from build123d import *

# Parameters (mm, degrees)
SKETCH1_W           = 76.2
SKETCH1_H           = 203.2
BOSS_EXTRUDE1_DEPTH = 6.35
SKETCH6_R           = 1.778
CUT_EXTRUDE4_DEPTH  = 6.35
SKETCH7_W           = 21.336
SKETCH7_H           = 38.1
BOSS_EXTRUDE2_DEPTH = 8.754615714
SKETCH8_R           = 1.778
CUT_EXTRUDE5_DEPTH  = 218.542707108
SKETCH9_W           = 44.45
SKETCH9_H           = 139.7
CUT_EXTRUDE6_DEPTH  = 3.175
CHAMFER1_SIZE       = 10


with BuildPart() as part:
    # Sketch1 → Boss-Extrude1 (new body)
    with BuildSketch(Plane.XY):
        with Locations((38.1, 101.6)):
            Rectangle(SKETCH1_W, SKETCH1_H)
    extrude(amount=BOSS_EXTRUDE1_DEPTH)

    # Sketch6 → Cut-Extrude4 (cut)
    with BuildSketch(Plane(origin=(0, 0, 0), x_dir=(-1, 0, 0), z_dir=(0, 0, -1))):
        with Locations((-63.5, 6.35)):
            Circle(SKETCH6_R)
        with Locations((-12.7, 6.35)):
            Circle(SKETCH6_R)
        with Locations((-6.35, 177.8)):
            Circle(SKETCH6_R)
        with Locations((-6.35, 25.4)):
            Circle(SKETCH6_R)
        with Locations((-69.85, 25.4)):
            Circle(SKETCH6_R)
        with Locations((-69.85, 177.8)):
            Circle(SKETCH6_R)
        with Locations((-63.5, 196.85)):
            Circle(SKETCH6_R)
        with Locations((-12.7, 196.85)):
            Circle(SKETCH6_R)
        with Locations((-6.35, 101.6)):
            Circle(SKETCH6_R)
        with Locations((-69.85, 101.6)):
            Circle(SKETCH6_R)
    extrude(amount=-CUT_EXTRUDE4_DEPTH, mode=Mode.SUBTRACT)

    # Sketch7 → Boss-Extrude2 (add)
    with BuildSketch(Plane.XY.offset(6.35)):
        with Locations((38.1, 19.05)):
            Rectangle(SKETCH7_W, SKETCH7_H)
    extrude(amount=BOSS_EXTRUDE2_DEPTH)

    # Sketch8 → Cut-Extrude5 (cut, through all)
    with BuildSketch(Plane.XY.offset(15.104615714)):
        with Locations((34.1503, 5.5753)):
            Circle(SKETCH8_R)
        with Locations((42.0497, 5.5753)):
            Circle(SKETCH8_R)
        with Locations((42.0497, 32.5247)):
            Circle(SKETCH8_R)
        with Locations((34.1503, 32.5247)):
            Circle(SKETCH8_R)
        with Locations((38.1, 19.05)):
            Circle(SKETCH8_R)
    extrude(amount=-CUT_EXTRUDE5_DEPTH, mode=Mode.SUBTRACT)

    # Sketch9 → Cut-Extrude6 (cut)
    with BuildSketch(Plane.XY.offset(6.35)):
        with Locations((38.1, 120.65)):
            Rectangle(SKETCH9_W, SKETCH9_H)
    extrude(amount=-CUT_EXTRUDE6_DEPTH, mode=Mode.SUBTRACT)

    # Chamfer1
    # the kernel refuses this chamfer: 10 mm, written as the material it adds along each edge
    with BuildSketch(Plane(origin=(27.432, 38.1, 6.35), x_dir=(-0.9996219169112968, 0, -0.027495876610586403), z_dir=(0, -1, 0))) as chamfer1_piece_1_section:
        Polygon((CHAMFER1_SIZE * 0.999621916911, -CHAMFER1_SIZE * 0.0274958766106), (-CHAMFER1_SIZE * 0.0274958766106, -CHAMFER1_SIZE * 0.999621916911), (0, 0), align=None)
    chamfer1_piece_1 = extrude(amount=38.1, mode=Mode.PRIVATE)
    chamfer1_piece_1 = split(chamfer1_piece_1, bisect_by=Plane(origin=(24.052510744, 19.05, 15.104615714), z_dir=(0, 0, -1)), keep=Keep.TOP, mode=Mode.PRIVATE)
    add(chamfer1_piece_1)
    with BuildSketch(Plane(origin=(48.768, 38.1, 6.35), x_dir=(0, 0.9996219169112968, -0.027495876610586403), z_dir=(-1, 0, 0))) as chamfer1_piece_2_section:
        Polygon((CHAMFER1_SIZE * 0.999621916911, -CHAMFER1_SIZE * 0.0274958766106), (-CHAMFER1_SIZE * 0.0274958766106, -CHAMFER1_SIZE * 0.999621916911), (0, 0), align=None)
    chamfer1_piece_2 = extrude(amount=21.336, mode=Mode.PRIVATE)
    chamfer1_piece_2 = split(chamfer1_piece_2, bisect_by=Plane(origin=(38.1, 41.479489256, 15.104615714), z_dir=(0, 0, -1)), keep=Keep.TOP, mode=Mode.PRIVATE)
    add(chamfer1_piece_2)
    with BuildSketch(Plane(origin=(48.768, 0, 6.35), x_dir=(0.9996219169112968, 0, -0.027495876610586403), z_dir=(0, 1, 0))) as chamfer1_piece_3_section:
        Polygon((CHAMFER1_SIZE * 0.999621916911, -CHAMFER1_SIZE * 0.0274958766106), (-CHAMFER1_SIZE * 0.0274958766106, -CHAMFER1_SIZE * 0.999621916911), (0, 0), align=None)
    chamfer1_piece_3 = extrude(amount=38.1, mode=Mode.PRIVATE)
    chamfer1_piece_3 = split(chamfer1_piece_3, bisect_by=Plane(origin=(52.147489256, 19.05, 15.104615714), z_dir=(0, 0, -1)), keep=Keep.TOP, mode=Mode.PRIVATE)
    add(chamfer1_piece_3)
    with BuildSketch(Plane(origin=(27.432, 63.81682988, 6.35), x_dir=(-0.9996219169112968, 0, -0.027495876610586403), z_dir=(0, -1, 0))) as chamfer1_piece_4a_section:
        Polygon((CHAMFER1_SIZE * 0.999621916911, -CHAMFER1_SIZE * 0.0274958766106), (-CHAMFER1_SIZE * 0.0274958766106, -CHAMFER1_SIZE * 0.999621916911), (0, 0), align=None)
    chamfer1_piece_4a = extrude(amount=63.81682988, mode=Mode.PRIVATE)
    chamfer1_piece_4a = split(chamfer1_piece_4a, bisect_by=Plane(origin=(24.052510744, 50.8, 9.492641484), z_dir=(0, -1, 0)), keep=Keep.TOP, mode=Mode.PRIVATE)
    chamfer1_piece_4a = split(chamfer1_piece_4a, bisect_by=Plane(origin=(24.052510744, 38.1, 9.492641484), z_dir=(0, 1, 0)), keep=Keep.TOP, mode=Mode.PRIVATE)
    chamfer1_piece_4a = split(chamfer1_piece_4a, bisect_by=Plane(origin=(24.052510744, 44.45, 15.104615714), z_dir=(0, 0, -1)), keep=Keep.TOP, mode=Mode.PRIVATE)
    with BuildSketch(Plane(origin=(48.768, 38.1, 6.35), x_dir=(0, 0.9996219169112968, -0.027495876610586403), z_dir=(-1, 0, 0))) as chamfer1_piece_4b_section:
        Polygon((CHAMFER1_SIZE * 0.999621916911, -CHAMFER1_SIZE * 0.0274958766106), (-CHAMFER1_SIZE * 0.0274958766106, -CHAMFER1_SIZE * 0.999621916911), (0, 0), align=None)
    chamfer1_piece_4b = extrude(amount=47.05282988, mode=Mode.PRIVATE)
    chamfer1_piece_4b = split(chamfer1_piece_4b, bisect_by=Plane(origin=(27.432, 41.479489256, 9.492641484), z_dir=(-1, 0, 0)), keep=Keep.TOP, mode=Mode.PRIVATE)
    chamfer1_piece_4b = split(chamfer1_piece_4b, bisect_by=Plane(origin=(14.57358506, 41.479489256, 15.104615714), z_dir=(0, 0, -1)), keep=Keep.TOP, mode=Mode.PRIVATE)
    chamfer1_piece_4 = chamfer1_piece_4a & chamfer1_piece_4b
    add(chamfer1_piece_4)
    with BuildSketch(Plane(origin=(74.48482988, 38.1, 6.35), x_dir=(0, 0.9996219169112968, -0.027495876610586403), z_dir=(-1, 0, 0))) as chamfer1_piece_5a_section:
        Polygon((CHAMFER1_SIZE * 0.999621916911, -CHAMFER1_SIZE * 0.0274958766106), (-CHAMFER1_SIZE * 0.0274958766106, -CHAMFER1_SIZE * 0.999621916911), (0, 0), align=None)
    chamfer1_piece_5a = extrude(amount=47.05282988, mode=Mode.PRIVATE)
    chamfer1_piece_5a = split(chamfer1_piece_5a, bisect_by=Plane(origin=(61.62641494, 41.479489256, 15.104615714), z_dir=(0, 0, -1)), keep=Keep.TOP, mode=Mode.PRIVATE)
    chamfer1_piece_5a = split(chamfer1_piece_5a, bisect_by=Plane(origin=(48.768, 41.479489256, 9.492641484), z_dir=(1, 0, 0)), keep=Keep.TOP, mode=Mode.PRIVATE)
    with BuildSketch(Plane(origin=(48.768, 0, 6.35), x_dir=(0.9996219169112968, 0, -0.027495876610586403), z_dir=(0, 1, 0))) as chamfer1_piece_5b_section:
        Polygon((CHAMFER1_SIZE * 0.999621916911, -CHAMFER1_SIZE * 0.0274958766106), (-CHAMFER1_SIZE * 0.0274958766106, -CHAMFER1_SIZE * 0.999621916911), (0, 0), align=None)
    chamfer1_piece_5b = extrude(amount=63.81682988, mode=Mode.PRIVATE)
    chamfer1_piece_5b = split(chamfer1_piece_5b, bisect_by=Plane(origin=(52.147489256, 50.8, 9.492641484), z_dir=(0, -1, 0)), keep=Keep.TOP, mode=Mode.PRIVATE)
    chamfer1_piece_5b = split(chamfer1_piece_5b, bisect_by=Plane(origin=(52.147489256, 44.45, 15.104615714), z_dir=(0, 0, -1)), keep=Keep.TOP, mode=Mode.PRIVATE)
    chamfer1_piece_5b = split(chamfer1_piece_5b, bisect_by=Plane(origin=(52.147489256, 38.1, 9.492641484), z_dir=(0, 1, 0)), keep=Keep.TOP, mode=Mode.PRIVATE)
    chamfer1_piece_5 = chamfer1_piece_5a & chamfer1_piece_5b
    add(chamfer1_piece_5)


solid = part.part
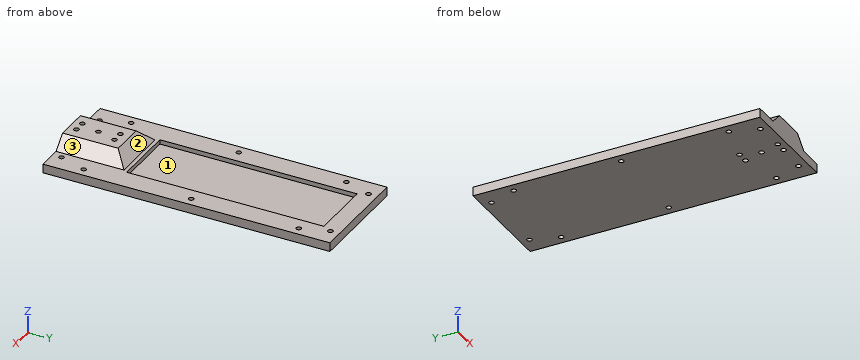
Work out the finished part from the listing and answer in its coordinate system (mm). Face numbers are marked on the shaded views. Round coordinates to 2 decimals unless told otherwise and drop trailing zeros. Write each loop counter-clockwise with the first axis right and the second up, starting at its lowest first coordinate (ties: lowest second). Pieces come first, ordered by that corner, then holes. Notation, with made-up numbers: (51.5, 84.25) - (89.5, 84.25) arc R28 cw to (89.5, 123.25) - close; hole circle Ø8 at (-4.5, 7). An arc over 180 degrees is marked (long way). Answer in a Markdown table with one row per item. Add a question column.
1. Given pin 1 (4 mm diameter, centred on x = 45.5, z = 8.5, fed in from +Y); pin 2 (1.5 mm diameter, centred on x = 54.5, z = 8.5, fed in from -Y), each flat-ended and moving along its own axis, determine where each tip first touches the part or whether it passes through.
2. Find the intervals of material crossed by line 1 along Y through (x, z) = (6.35, 4); line 2 along X through (y, z) = (177.8, 2.25); line 3 along X through (y, z) = (131, 4.5) (3 decimals), in increasing order. Write a range as from..to.
3. A cutting plane is placed at A-A, the plane x = 38.1. Determine the outline of the cut face in (y, z) (3 decimals), and give its area (3 significant figures).
4. The mould has two halves that part along Y. Classify the marked faces 1, 2 and 3: +Y half, -Y half, draft (parallel to the pull), parting line (faces both ways), or undercut.
5. A cutting plane is placed at D-D, the plane y = 15.5. Determine the outline of the cut face in (x, z), and give its area (3 significant figures).
6. A cutting plane is placed at B-B, the plane y = 177.8. Determine the outline of the cut face in (x, z) (3 decimals).
7. A cutting plane is placed at C-C, the plane x = 12.7. Determine the outline of the cut face in (y, z), and give its area (3 significant figures).
Worked out:
| question | item | result |
|---|---|---|
| 1 | pin 1 | y = 47.95 |
| 1 | pin 2 | y = 0 |
| 2 | line 1 | 0..23.62, 27.18..99.82, 103.38..176.02, 179.58..203.2 |
| 2 | line 2 | 0..4.57, 8.13..68.07, 71.63..76.2 |
| 2 | line 3 | 0..15.875, 60.325..76.2 |
| 3 | outline | (0, 0) - (17.272, 0) - (17.272, 15.105) - (0, 15.105) - close; (20.828, 0) - (203.2, 0) - (203.2, 6.35) - (190.5, 6.35) - (190.5, 3.175) - (50.8, 3.175) - (50.8, 6.35) - (48.1, 6.35) - (39.345, 15.105) - (20.828, 15.105) - close |
| 3 | area | 1,180 mm^2 |
| 4 | face 1 | undercut |
| 4 | face 2 | +Y half |
| 4 | face 3 | draft |
| 5 | outline | (0, 0) - (76.2, 0) - (76.2, 6.35) - (58.77, 6.35) - (50.01, 15.1) - (26.19, 15.1) - (17.43, 6.35) - (0, 6.35) - close |
| 5 | area | 769 mm^2 |
| 6 | outline | (0, 0) - (4.572, 0) - (4.572, 6.35) - (0, 6.35) - close; (8.128, 0) - (68.072, 0) - (68.072, 6.35) - (60.325, 6.35) - (60.325, 3.175) - (15.875, 3.175) - (15.875, 6.35) - (8.128, 6.35) - close; (71.628, 0) - (76.2, 0) - (76.2, 6.35) - (71.628, 6.35) - close |
| 7 | outline | (0, 0) - (4.57, 0) - (4.57, 6.35) - (0, 6.35) - close; (8.13, 0) - (195.07, 0) - (195.07, 6.35) - (8.13, 6.35) - close; (198.63, 0) - (203.2, 0) - (203.2, 6.35) - (198.63, 6.35) - close |
| 7 | area | 1,250 mm^2 |
